Geometry: final body of the model. Coordinates: model frame, mm. Face numbers are marked on the shaded views. Round coordinates to 2 decimals unless told otherwise and drop trailing zeros. Loops run counter-clockwise (first coordinate to the right, second up) from the corner with the lowest first, then second, coordinate; pieces in that order, holes last. Notation, with made-up numbers: M 46,30 L 66,30 A12 ccw 66,44 Z; hole C 75.25,51.25 d10. An arc over 180 degrees is marked long. Answer as a JSON object with one key per item and string values.
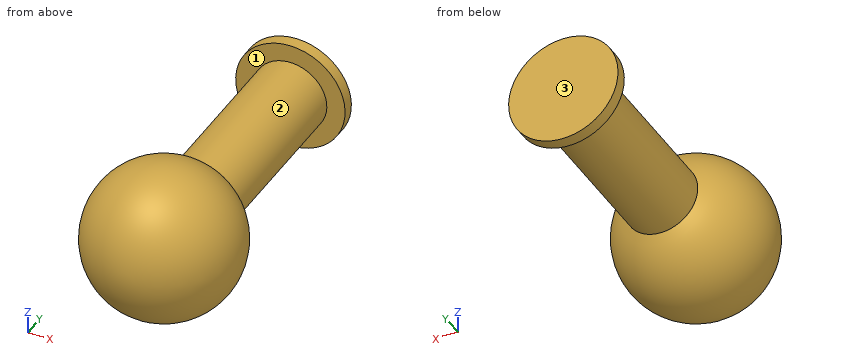
```python
from build123d import *

# Parameters (mm, degrees)
SKETCH2_R           = 7.62
BOSS_EXTRUDE1_DEPTH = 50.8
SKETCH3_R           = 11.43
BOSS_EXTRUDE2_DEPTH = 2.54


with BuildPart() as part:
    # Sketch1 → Revolve1 (revolve)
    with BuildSketch(Plane.XY):
        with BuildLine():
            Line((0, -15.875), (0, 15.875))
            ThreePointArc((0, 15.875), (15.875, 0), (0, -15.875))
        make_face()
    revolve(axis=Axis((0, -15.875, 0), (0, 1, 0)))

    # Sketch2 → Boss-Extrude1 (add)
    with BuildSketch(Plane(origin=(0, 0, 0), x_dir=(1, 0, 0), z_dir=(0, 1, 0))):
        with Locations(Location((0, 0, 0), (0, 0, 90))):
            Circle(SKETCH2_R)
    extrude(amount=BOSS_EXTRUDE1_DEPTH)

    # Sketch3 → Boss-Extrude2 (add)
    with BuildSketch(Plane(origin=(0, 50.8, 0), x_dir=(1, 0, 0), z_dir=(0, 1, 0))):
        with Locations(Location((0, 0, 0), (0, 0, 270))):
            Circle(SKETCH3_R)
    extrude(amount=BOSS_EXTRUDE2_DEPTH)


solid = part.part
```
1) Cut plane A-A on z = 0. Return the cut outline in (x, y) (3 decimals).
Geometry results:
{"outline": "M -11.43,50.8 L -7.62,50.8 L -7.62,13.927 A15.875 ccw long 7.62,13.927 L 7.62,50.8 L 11.43,50.8 L 11.43,53.34 L -11.43,53.34 Z"}
2) Cut plane B-B on x = 0. Return the cut outline in (y, z) (3 decimals), and give its area (3 significant figures).
Geometry results:
{"outline": "M 13.927,-7.62 L 50.8,-7.62 L 50.8,-11.43 L 53.34,-11.43 L 53.34,11.43 L 50.8,11.43 L 50.8,7.62 L 13.927,7.62 A15.875 ccw long Z", "area": "1,390 mm2"}
3) First-contact query: pin 1 (12 mm diameter, centred on y = 30.5, z = 12.5, fed in from -X); pin 2 (12 mm diameter, centred on y = 19.5, z = -3.5, fed in from +X); pin 3 (2 mm diameter, centred on x = -4.5, z = -1, fed in from -Y). Flat tips, straight axial feed; report the tip coordinate or a pass-through.
Geometry results:
{"pin 1": "x = -3.98", "pin 2": "x = 7.83", "pin 3": "y = -15.46"}
4) Pull-direction query (Y, two-part tool) for the marked faces 1, 2 and 3; classes: +Y half, -Y half, draft (parallel to the pull), parting line (faces both ways), or undercut.
Geometry results:
{"face 1": "undercut", "face 2": "undercut", "face 3": "+Y half"}
5) Cut plane C-C on y = 18.5. Return the cut outline in (x, z), and give its area (3 significant figures).
Geometry results:
{"outline": "C 0,0 d15.24", "area": "182 mm2"}
6) Cut plane D-D on x = -9.5. Return the cut outline in (y, z).
Geometry results:
{"outline": "C 0,0 d25.44; M 50.8,-6.36 L 53.34,-6.36 L 53.34,6.36 L 50.8,6.36 Z"}
7) Line query: probe 1 along Y at (x, z) = (-5, 7); probe 2 along Y at (x, z) = (-6, -4); probe 3 along Y at (x, z) = (11.5, -6). Output: solid intervals per line, ascending.
Geometry results:
{"probe 1": "-13.34 to 13.34, 50.8 to 53.34", "probe 2": "-14.14 to 53.34", "probe 3": "-9.15 to 9.15"}
